Input: part model. Units: mm. Frame: model coordinates. Face numbers are marked on the shaded views. Give positions to 0.01 mm unless a question says otherwise; leave off trailing zeros. Order: outer loops, then holes, each group sorted by start corner. A loop starts at its lowest first (then second) coordinate and runs counter-clockwise, first axis right, second up. Notation, with made-up numbers: (-17, 87.25) - (36, 87.25) arc R10 cw to (36, 104.25) - close; hole circle Ø2 at (-5, -30). An arc over 180 degrees is marked (long way). Answer in a Markdown table with one row per item. Add a question column.
1. Ray query, line 1 (Y direction, x = 8, z = 0); line 2 (Y direction, x = 21, z = 3.25); line 3 (X direction, y = 68.5, z = 0.5). Return the intervals inside material, ascending. Write a range as [from, to].
2. Section query B-B on z = 0. Return loops of the section in (x, y), and give its area (3 significant figures).
3. Contact query for flat-ended pins moving along their axis: pin 1 (1 mm diameter, centred on y = 63, z = -3.5, fed in from -X); pin 2 (6 mm diameter, centred on x = 72, z = 1.5, fed in from +Y); pin 3 (5 mm diameter, centred on y = 68.5, z = 0.5, fed in from -X). Output: stop coordinate, or through.
4. Section query A-A on z = -6. Return loops of the section in (x, y).
5. Mould query, pull axis Z, two halves, no side actions, for the marked faces 1 and 2. Classes: released by +Z, released by -Z, zero draft, split by the parting line, or undercut.
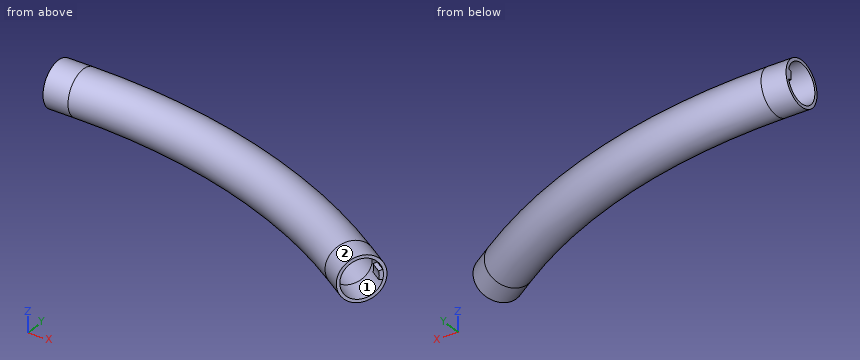
```python
from build123d import *

# Parameters (mm, degrees)
SKETCH3_R           = 9
SKETCH3_R_2         = 7.75
BOSS_EXTRUDE3_DEPTH = 5
BOSS_EXTRUDE4_START = -5
BOSS_EXTRUDE4_DEPTH = 5


with BuildPart() as part:
    # Sweep1: sweep along a path in Sketch2path
    with BuildLine(Plane.XY) as sweep1_path:
        Line((0, 100), (10, 100))
        ThreePointArc((10, 100), (80.430596643, 89.552607894), (144.795757594, 59.110153969))
        Line((144.795757594, 59.110153969), (153.110453717, 53.554451639))
    # Sketch3 → Sweep1 (sweep)
    with BuildSketch(Plane(origin=(0, 0, 0), x_dir=(0, 0, -1), z_dir=(1, 0, 0))):
        with Locations((0, 100)):
            Circle(SKETCH3_R)
        with Locations((0, 100)):
            Circle(SKETCH3_R_2, mode=Mode.SUBTRACT)
    sweep(path=sweep1_path.line)

    # Sketch8 → Boss-Extrude3 (add)
    with BuildSketch(Plane(origin=(81.112712966, -54.197782068, 0), x_dir=(0, 0, -1), z_dir=(0.8314696123025445, -0.5555702330196034, 0))):
        with BuildLine():
            Line((-1.617619032, 135.629546005), (-2.0058476, 137.078434745))
            ThreePointArc((-2.0058476, 137.078434745), (0, 137.342509591), (2.0058476, 137.078434745))
            Line((2.0058476, 137.078434745), (1.617619032, 135.629546005))
            ThreePointArc((1.617619032, 135.629546005), (0, 135.842509591), (-1.617619032, 135.629546005))
        make_face()
    extrude(amount=-BOSS_EXTRUDE3_DEPTH)

    # Sketch9 → Boss-Extrude4 (add)
    with BuildSketch(Plane.ZY.offset(BOSS_EXTRUDE4_START)):
        with BuildLine():
            Line((-1.617619032, 106.037036414), (-2.0058476, 107.485925154))
            ThreePointArc((-2.0058476, 107.485925154), (0, 107.75), (2.0058476, 107.485925154))
            Line((2.0058476, 107.485925154), (1.617619032, 106.037036414))
            ThreePointArc((1.617619032, 106.037036414), (0, 106.25), (-1.617619032, 106.037036414))
        make_face()
    extrude(amount=BOSS_EXTRUDE4_DEPTH)


solid = part.part
```
Answer:
| question | item | result |
|---|---|---|
| 1 | line 1 | y = [91, 92.25], [107.75, 109] |
| 1 | line 2 | y = [91.35, 92.71], [106.79, 108.15] |
| 1 | line 3 | x = [110.07, 112.96], [144.56, 146.87] |
| 2 | outline | (0, 91) - (10, 91) arc R233.63 cw to (139.8, 51.63) - (148.11, 46.07) - (148.8, 47.11) - (140.49, 52.67) arc R234.88 ccw to (10, 92.25) - (0, 92.25) - close; (0, 106.25) - (5, 106.25) - (5, 107.75) - (10, 107.75) arc R250.38 cw to (149.1, 65.55) - (153.26, 62.78) - (152.43, 61.53) - (156.58, 58.75) - (158.11, 61.04) - (149.8, 66.59) arc R251.63 ccw to (10, 109) - (0, 109) - close |
| 2 | area | 422 mm² |
| 3 | pin 1 | stops at x = 121.37 |
| 3 | pin 2 | stops at y = 101.93 |
| 3 | pin 3 | stops at x = 104.6 |
| 4 | outline | (0, 93.29) - (10, 93.29) arc R235.92 cw to (141.07, 53.53) - (149.38, 47.98) - (150.39, 49.48) - (142.07, 55.03) arc R237.72 ccw to (10, 95.09) - (0, 95.09) - close; (0, 104.91) - (10, 104.91) arc R247.53 cw to (147.52, 63.19) - (155.84, 57.63) - (156.84, 59.13) - (148.52, 64.69) arc R249.33 ccw to (10, 106.71) - (0, 106.71) - close |
| 5 | face 1 | undercut |
| 5 | face 2 | split by the parting line |
